```python
from build123d import *

# Parameters (mm, degrees)
BOX_W        = 190
BOX_H        = 95
BOX_DEPTH    = 2
BOX001_W     = 186
BOX001_H     = 89
BOX001_DEPTH = 10
BOX002_W     = 184
BOX002_H     = 87
BOX002_DEPTH = 10
BOX003_W     = 160
BOX003_H     = 89
BOX003_DEPTH = 10


with BuildPart() as part:
    # Box → Box (join)
    with BuildSketch(Plane.XY):
        with Locations((95, 47.5)):
            Rectangle(BOX_W, BOX_H)
    extrude(amount=BOX_DEPTH)

    # Box001 → Box001 (join)
    with BuildSketch(Plane(origin=(2, 2, 0), x_dir=(1, 0, 0), z_dir=(0, 0, 1))):
        with Locations((93, 44.5)):
            Rectangle(BOX001_W, BOX001_H)
    extrude(amount=BOX001_DEPTH)

    # Box002 → Box002 (cut)
    with BuildSketch(Plane(origin=(3, 3, 0), x_dir=(1, 0, 0), z_dir=(0, 0, 1))):
        with Locations((92, 43.5)):
            Rectangle(BOX002_W, BOX002_H)
    extrude(amount=BOX002_DEPTH, mode=Mode.SUBTRACT)

    # Box003 → Box003 (cut)
    with BuildSketch(Plane(origin=(13, 2, 2), x_dir=(1, 0, 0), z_dir=(0, 0, 1))):
        with Locations((80, 44.5)):
            Rectangle(BOX003_W, BOX003_H)
    extrude(amount=BOX003_DEPTH, mode=Mode.SUBTRACT)


solid = part.part
```
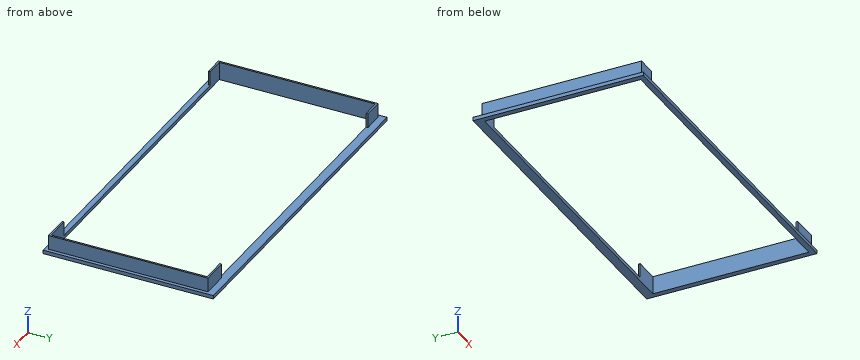
CAD build for the part. Positions are in the model's coordinates, mm. Round coordinates to 2 decimals unless told otherwise and drop trailing zeros. Loops run counter-clockwise (first coordinate to the right, second up) from the corner with the lowest first, then second, coordinate; pieces in that order, holes last. Notation, with made-up numbers: M -17,7 L -3,7 A30 cw -3,36 Z; hole C -14,-31 d3. An arc over 180 degrees is marked long. Use a Markdown table: item, result. Add a question column.
(1) Cut at C-C (x = 135). Give the cut face in (y, z), and give its area (3 significant figures).
(2) Flat gauge pins, fed straight in: pin 1 (3 mm diameter, centred on y = 27.5, z = 2.5, fed in from +X); pin 2 (0.5 mm diameter, centred on y = 90.5, z = 4.5, fed in from -X); pin 3 (4 mm diameter, centred on x = 180.5, z = 7, fed in from -Y); pin 4 (0.8 mm diameter, centred on y = 2.5, z = 7.5, fed in from +X). Where does each tip first touch, or does it go through?
(3) Cut at B-B (z = 5.5). Give the cut face in (x, y), and give its area (3 significant figures).
(4) Cut at A-A (y = 61). Give the cut face in (x, z).
(5) Drill centre lines: line 1 (X direction, y = 8, z = 6.25); line 2 (Y direction, x = 182, z = 4.25); line 3 (X direction, y = 75.5, z = 1.25). Where is each one in solid material? Low to high.
Geometry says:
| question | item | result |
|---|---|---|
| 1 | outline | M 0,0 L 3,0 L 3,2 L 0,2 Z; M 90,0 L 95,0 L 95,2 L 90,2 Z |
| 1 | area | 16.0 mm² |
| 2 | pin 1 | stops at x = 190 |
| 2 | pin 2 | stops at x = 2 |
| 2 | pin 3 | stops at y = 2 |
| 2 | pin 4 | stops at x = 188 |
| 3 | outline | M 2,2 L 13,2 L 13,3 L 3,3 L 3,90 L 13,90 L 13,91 L 2,91 Z; M 173,2 L 188,2 L 188,91 L 173,91 L 173,90 L 187,90 L 187,3 L 173,3 Z |
| 3 | area | 226 mm² |
| 4 | outline | M 0,0 L 3,0 L 3,10 L 2,10 L 2,2 L 0,2 Z; M 187,0 L 190,0 L 190,2 L 188,2 L 188,10 L 187,10 Z |
| 5 | line 1 | x = 2 to 3, 187 to 188 |
| 5 | line 2 | y = 2 to 3, 90 to 91 |
| 5 | line 3 | x = 0 to 3, 187 to 190 |
